Part model, mm, in its own coordinate system. Face numbers are marked on the shaded views. A direction names the side the tool comes from. Give positions to 0.01 mm unless a question says otherwise; leave off trailing zeros. Order: outer loops, then holes, each group sorted by start corner. A loop starts at its lowest first (then second) coordinate and runs counter-clockwise, first axis right, second up. Notation, with made-up numbers: (26.5, 46.5) -> (44.5, 46.5) arc R24 cw to (44.5, 81.5) -> close; hole circle Ø10 at (7.5, 78). An arc over 180 degrees is marked (long way). Write item = value, one per line. Start each with the question number.
(1) Two-plate mould, pull along X, no slides. Class the marked faces 3, 4 and 5: pulls with the +X half, pulls with the -X half, needs draft (parallel to the pull), parting line crosses it, or undercut.
(2) Flat gauge pins, fed straight in: pin 1 (5.5 mm diameter, centred on x = 18.5, y = 4.5, fed in from -Z); pin 2 (4.5 mm diameter, centred on x = 15, z = 25, fed in from +Y); pin 3 (2 mm diameter, centred on y = 4, z = 10, fed in from +X); pin 4 (1.5 mm diameter, centred on y = 3, z = 26.5, fed in from -X). Where does each tip first touch, or does it go through?
(3) Probe line 1 along Z through (x, y) = (15, 7.75); line 2 along Z through (x, y) = (15.5, 8.25); line 3 along X through (y, z) = (3.75, 23.75). List the from-to ranges inside material, lowest first. Write a range as from..to.
(4) Saw through at A-A, the plane y = 0.75. List the corners of the cut face in (x, z).
(5) Which spindle directions (+Z, -Z, +X, -X, +Y, -Y) get a long thin tool onto all of the face, cutting with end or side? Do the marked faces 1 and 2. Say none if no direction does.
(6) Saw through at D-D, the plane z = 9.75. List the corners of the cut face in (x, y).
(7) Saw through at B-B, the plane z = 25. List the corners of the cut face in (x, y), then the cut area to 3 significant figures.
(8) Saw through at C-C, the plane x = 15.5. List the corners of the cut face in (y, z).
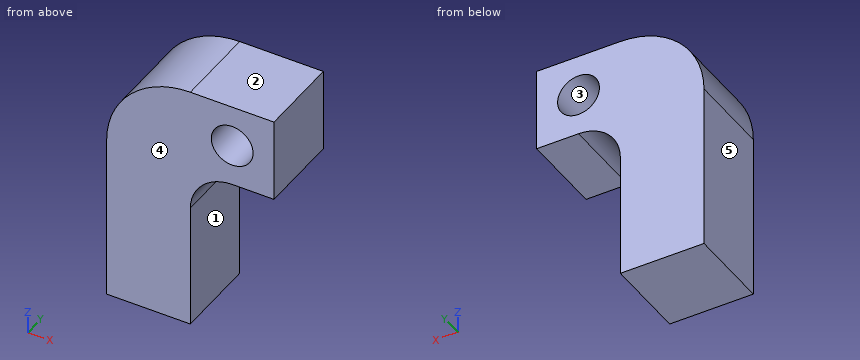
from build123d import *

# Parameters (mm, degrees)
BOSS_EXTRUDE1_DEPTH = 10
FILLET1_R           = 5
FILLET1_2_R         = 10
SKETCH3_R           = 2.5
CUT_EXTRUDE1_DEPTH  = 11


with BuildPart() as part:
    # Sketch2 → Boss-Extrude1 (new body)
    with BuildSketch(Plane(origin=(0, 0, 0), x_dir=(1, 0, 0), z_dir=(0, 1, 0))):
        Polygon((10, 0), (0, 0), (0, -30), (5, -30), (20, -30), (20, -20), (10, -20), align=None)
    extrude(amount=BOSS_EXTRUDE1_DEPTH)

    # Fillet1
    fillet1_edges = [part.edges().sort_by_distance(p)[0] for p in [
        (10, 5, 20),
    ]]
    fillet(fillet1_edges, radius=FILLET1_R)

    # Fillet1 2
    fillet1_2_edges = [part.edges().sort_by_distance(p)[0] for p in [
        (0, 5, 30),
    ]]
    fillet(fillet1_2_edges, radius=FILLET1_2_R)

    # Sketch3 → Cut-Extrude1 (cut, through all)
    with BuildSketch(Plane(origin=(0, 10, 0), x_dir=(1, 0, 0), z_dir=(0, 1, 0))):
        with Locations((15, -25)):
            Circle(SKETCH3_R)
    extrude(amount=-CUT_EXTRUDE1_DEPTH, mode=Mode.SUBTRACT)


solid = part.part
Results list:
q1.face_3 = undercut
q1.face_4 = needs draft
q1.face_5 = pulls with the -X half
q2.pin_1 = 20
q2.pin_2 = through
q2.pin_3 = 10
q2.pin_4 = 1.82
q3.line_1 = 20..22.5, 27.5..30
q3.line_2 = 20..22.55, 27.45..30
q3.line_3 = 0.73..12.83, 17.17..20
q4.outline = (0, 0) -> (10, 0) -> (10, 15) arc R5 cw to (15, 20) -> (20, 20) -> (20, 30) -> (10, 30) arc R10 ccw to (0, 20) -> close; hole circle Ø5 at (15, 25)
q5.face_1 = -Z, +X, +Y, -Y
q5.face_2 = +Z, +X, -X, +Y, -Y
q6.outline = (0, 0) -> (10, 0) -> (10, 10) -> (0, 10) -> close
q7.outline = (1.34, 0) -> (12.5, 0) -> (12.5, 10) -> (1.34, 10) -> close; (17.5, 0) -> (20, 0) -> (20, 10) -> (17.5, 10) -> close
q7.area = 137 mm^2
q8.outline = (0, 20) -> (10, 20) -> (10, 22.55) -> (0, 22.55) -> close; (0, 27.45) -> (10, 27.45) -> (10, 30) -> (0, 30) -> close
